Design review of the part shown in the three views and the two pictorial views. Dimensions are in mm from the part's minimum x, y and z. Coordinates: 2 decimals unless noted, no trailing zeros. Loops run counter-clockwise (first coordinate to the right, second up) from the corner with the lowest first, then second, coordinate; pieces in that order, holes last. Notation, with made-up numbers: (60, -29) -> (67, -29) arc R25 ccw to (67, 10) -> close; hole circle Ø4 at (66, 69.5). An arc over 180 degrees is marked (long way). Answer in a Markdown table with one row per item.
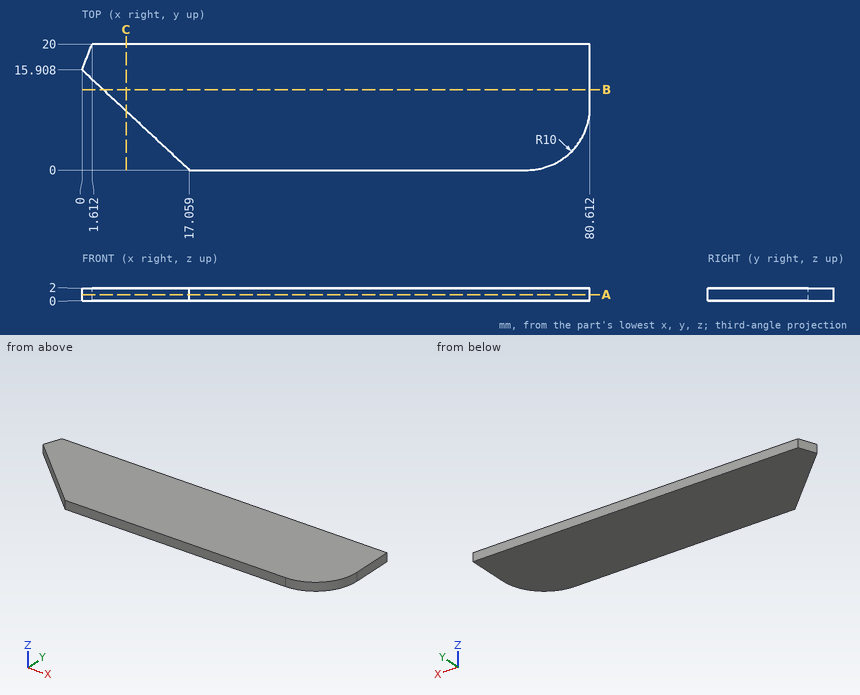
Item 1: Take a section at C-C, the plane x = 7. State the section outline as (y, z) points.
Worked answers:
| item | result |
|---|---|
| outline | (9.38, 0) -> (20, 0) -> (20, 2) -> (9.38, 2) -> close |
Item 2: Insertion check: pin 1 (1 mm diameter, centred on y = 8, z = 0.5, fed in from +X). The pin has a flat end and moves straight along its axis. Give the tip position at first contact, or say it passes through.
Worked answers:
| item | result |
|---|---|
| pin 1 | x = 80.5 |
Item 3: Take a section at A-A, the plane z = 0.95. State the section outline as (x, y) points, and give its area (3 significant figures).
Worked answers:
| item | result |
|---|---|
| outline | (0, 15.91) -> (17.06, 0) -> (70.61, 0) arc R10 ccw to (80.61, 10) -> (80.61, 20) -> (1.61, 20) -> close |
| area | 1,450 mm² |
Item 4: For L1, parallel to X at y = 4, z = 0.8; L2, parallel to Y at x = 73.5, z = 1.4; L3, parallel to X at y = 17.75, z = 1.3 (1 decimal), list the stretches that pass through material, from the lowest coordinate up.
Worked answers:
| item | result |
|---|---|
| L1 | 12.77 to 78.61 |
| L2 | 0.43 to 20 |
| L3 | 0.7 to 80.6 |
Item 5: Take a section at B-B, the plane y = 12.75. State the section outline as (x, z) points.
Worked answers:
| item | result |
|---|---|
| outline | (3.39, 0) -> (80.61, 0) -> (80.61, 2) -> (3.39, 2) -> close |
